```python
from build123d import *

# Parameters (mm, degrees)
ESBO_O1_W                = 72
ESBO_O1_H                = 110
RESSALTO_EXTRUS_O1_DEPTH = 5
ESBO_O2_W                = 51
ESBO_O2_H                = 72
CORTE_EXTRUS_O1_DEPTH    = 4
CHANFRO1_SIZE            = 1.5
CHANFRO1_SIZE_2          = 4
CORTE_EXTRUS_O2_DEPTH    = 66.924198895
CORTE_EXTRUS_O3_DEPTH    = 66.924198895
CORTE_EXTRUS_O4_DEPTH    = 3
CORTE_EXTRUS_O5_DEPTH    = 3
ESBO_O7_W                = 31
ESBO_O7_H                = 44
RESSALTO_EXTRUS_O2_DEPTH = 17
ESBO_O8_W                = 28
ESBO_O8_H                = 42
CORTE_EXTRUS_O6_DEPTH    = 70.318107302
ESBO_O9_W                = 3
ESBO_O9_H                = 1
RESSALTO_EXTRUS_O3_DEPTH = 10
FILETE1_R                = 2


with BuildPart() as part:
    # Esboço1 → Ressalto-extrusão1 (new body)
    with BuildSketch(Plane.XY):
        Rectangle(ESBO_O1_W, ESBO_O1_H)
    extrude(amount=RESSALTO_EXTRUS_O1_DEPTH)

    # Esboço2 → Corte-extrusão1 (cut)
    with BuildSketch(Plane.XY.offset(5)):
        Rectangle(ESBO_O2_W, ESBO_O2_H)
    extrude(amount=-CORTE_EXTRUS_O1_DEPTH, mode=Mode.SUBTRACT)

    # Chanfro1
    # the kernel refuses this chamfer: 4, 1.5 mm, written as the material it takes off along each edge
    with BuildSketch(Plane(origin=(-25.5, -36, 5), x_dir=(0, -0.9953980532473654, 0.09582648689874358), z_dir=(1, 0, 0))) as chanfro1_piece_1_section:
        Polygon((CHANFRO1_SIZE * 0.995398053247, CHANFRO1_SIZE * 0.0958264868987), (-CHANFRO1_SIZE_2 * 0.0958264868987, CHANFRO1_SIZE_2 * 0.995398053247), (0, 0), align=None)
    chanfro1_piece_1 = extrude(amount=51, mode=Mode.PRIVATE)
    chanfro1_piece_1 = split(chanfro1_piece_1, bisect_by=Plane(origin=(0, -36.465264147, 1), z_dir=(0, 0, 1)), keep=Keep.TOP, mode=Mode.PRIVATE)
    add(chanfro1_piece_1, mode=Mode.SUBTRACT)
    with BuildSketch(Plane(origin=(-25.5, 36, 5), x_dir=(-0.9953980532473654, 0, 0.09582648689874379), z_dir=(0, -1, 0))) as chanfro1_piece_2_section:
        Polygon((CHANFRO1_SIZE * 0.995398053247, CHANFRO1_SIZE * 0.0958264868987), (-CHANFRO1_SIZE_2 * 0.0958264868987, CHANFRO1_SIZE_2 * 0.995398053247), (0, 0), align=None)
    chanfro1_piece_2 = extrude(amount=72, mode=Mode.PRIVATE)
    chanfro1_piece_2 = split(chanfro1_piece_2, bisect_by=Plane(origin=(-25.965264147, 0, 1), z_dir=(0, 0, 1)), keep=Keep.TOP, mode=Mode.PRIVATE)
    add(chanfro1_piece_2, mode=Mode.SUBTRACT)
    with BuildSketch(Plane(origin=(25.5, -36, 5), x_dir=(0.9953980532473654, 0, 0.09582648689874379), z_dir=(0, 1, 0))) as chanfro1_piece_3_section:
        Polygon((CHANFRO1_SIZE * 0.995398053247, CHANFRO1_SIZE * 0.0958264868987), (-CHANFRO1_SIZE_2 * 0.0958264868987, CHANFRO1_SIZE_2 * 0.995398053247), (0, 0), align=None)
    chanfro1_piece_3 = extrude(amount=72, mode=Mode.PRIVATE)
    chanfro1_piece_3 = split(chanfro1_piece_3, bisect_by=Plane(origin=(25.965264147, 0, 1), z_dir=(0, 0, 1)), keep=Keep.TOP, mode=Mode.PRIVATE)
    add(chanfro1_piece_3, mode=Mode.SUBTRACT)
    with BuildSketch(Plane(origin=(25.5, 36, 5), x_dir=(0, 0.9953980532473654, 0.09582648689874358), z_dir=(-1, 0, 0))) as chanfro1_piece_4_section:
        Polygon((CHANFRO1_SIZE * 0.995398053247, CHANFRO1_SIZE * 0.0958264868987), (-CHANFRO1_SIZE_2 * 0.0958264868987, CHANFRO1_SIZE_2 * 0.995398053247), (0, 0), align=None)
    chanfro1_piece_4 = extrude(amount=51, mode=Mode.PRIVATE)
    chanfro1_piece_4 = split(chanfro1_piece_4, bisect_by=Plane(origin=(0, 36.465264147, 1), z_dir=(0, 0, 1)), keep=Keep.TOP, mode=Mode.PRIVATE)
    add(chanfro1_piece_4, mode=Mode.SUBTRACT)
    with BuildSketch(Plane(origin=(-35.875482322, -36, 5), x_dir=(0, -0.9953980532473654, 0.09582648689874358), z_dir=(1, 0, 0))) as chanfro1_piece_5a_section:
        Polygon((CHANFRO1_SIZE * 0.995398053247, CHANFRO1_SIZE * 0.0958264868987), (-CHANFRO1_SIZE_2 * 0.0958264868987, CHANFRO1_SIZE_2 * 0.995398053247), (0, 0), align=None)
    chanfro1_piece_5a = extrude(amount=61.375482322, mode=Mode.PRIVATE)
    chanfro1_piece_5a = split(chanfro1_piece_5a, bisect_by=Plane(origin=(-25.5, -36.465264147, 3.645492171), z_dir=(-1, 0, 0)), keep=Keep.TOP, mode=Mode.PRIVATE)
    chanfro1_piece_5a = split(chanfro1_piece_5a, bisect_by=Plane(origin=(-30.687741161, -36.465264147, 1), z_dir=(0, 0, 1)), keep=Keep.TOP, mode=Mode.PRIVATE)
    with BuildSketch(Plane(origin=(-25.5, 36, 5), x_dir=(-0.9953980532473654, 0, 0.09582648689874379), z_dir=(0, -1, 0))) as chanfro1_piece_5b_section:
        Polygon((CHANFRO1_SIZE * 0.995398053247, CHANFRO1_SIZE * 0.0958264868987), (-CHANFRO1_SIZE_2 * 0.0958264868987, CHANFRO1_SIZE_2 * 0.995398053247), (0, 0), align=None)
    chanfro1_piece_5b = extrude(amount=82.375482322, mode=Mode.PRIVATE)
    chanfro1_piece_5b = split(chanfro1_piece_5b, bisect_by=Plane(origin=(-25.965264147, -36, 3.645492171), z_dir=(0, -1, 0)), keep=Keep.TOP, mode=Mode.PRIVATE)
    chanfro1_piece_5b = split(chanfro1_piece_5b, bisect_by=Plane(origin=(-25.965264147, -41.187741161, 1), z_dir=(0, 0, 1)), keep=Keep.TOP, mode=Mode.PRIVATE)
    chanfro1_piece_5 = chanfro1_piece_5a & chanfro1_piece_5b
    add(chanfro1_piece_5, mode=Mode.SUBTRACT)
    with BuildSketch(Plane(origin=(-25.5, -36, 5), x_dir=(0, -0.9953980532473654, 0.09582648689874358), z_dir=(1, 0, 0))) as chanfro1_piece_6a_section:
        Polygon((CHANFRO1_SIZE * 0.995398053247, CHANFRO1_SIZE * 0.0958264868987), (-CHANFRO1_SIZE_2 * 0.0958264868987, CHANFRO1_SIZE_2 * 0.995398053247), (0, 0), align=None)
    chanfro1_piece_6a = extrude(amount=61.375482322, mode=Mode.PRIVATE)
    chanfro1_piece_6a = split(chanfro1_piece_6a, bisect_by=Plane(origin=(25.5, -36.465264147, 3.645492171), z_dir=(1, 0, 0)), keep=Keep.TOP, mode=Mode.PRIVATE)
    chanfro1_piece_6a = split(chanfro1_piece_6a, bisect_by=Plane(origin=(30.687741161, -36.465264147, 1), z_dir=(0, 0, 1)), keep=Keep.TOP, mode=Mode.PRIVATE)
    with BuildSketch(Plane(origin=(25.5, -46.375482322, 5), x_dir=(0.9953980532473654, 0, 0.09582648689874379), z_dir=(0, 1, 0))) as chanfro1_piece_6b_section:
        Polygon((CHANFRO1_SIZE * 0.995398053247, CHANFRO1_SIZE * 0.0958264868987), (-CHANFRO1_SIZE_2 * 0.0958264868987, CHANFRO1_SIZE_2 * 0.995398053247), (0, 0), align=None)
    chanfro1_piece_6b = extrude(amount=82.375482322, mode=Mode.PRIVATE)
    chanfro1_piece_6b = split(chanfro1_piece_6b, bisect_by=Plane(origin=(25.965264147, -36, 3.645492171), z_dir=(0, -1, 0)), keep=Keep.TOP, mode=Mode.PRIVATE)
    chanfro1_piece_6b = split(chanfro1_piece_6b, bisect_by=Plane(origin=(25.965264147, -41.187741161, 1), z_dir=(0, 0, 1)), keep=Keep.TOP, mode=Mode.PRIVATE)
    chanfro1_piece_6 = chanfro1_piece_6a & chanfro1_piece_6b
    add(chanfro1_piece_6, mode=Mode.SUBTRACT)
    with BuildSketch(Plane(origin=(25.5, 36, 5), x_dir=(0, 0.9953980532473654, 0.09582648689874358), z_dir=(-1, 0, 0))) as chanfro1_piece_7a_section:
        Polygon((CHANFRO1_SIZE * 0.995398053247, CHANFRO1_SIZE * 0.0958264868987), (-CHANFRO1_SIZE_2 * 0.0958264868987, CHANFRO1_SIZE_2 * 0.995398053247), (0, 0), align=None)
    chanfro1_piece_7a = extrude(amount=61.375482322, mode=Mode.PRIVATE)
    chanfro1_piece_7a = split(chanfro1_piece_7a, bisect_by=Plane(origin=(-25.5, 36.465264147, 3.645492171), z_dir=(-1, 0, 0)), keep=Keep.TOP, mode=Mode.PRIVATE)
    chanfro1_piece_7a = split(chanfro1_piece_7a, bisect_by=Plane(origin=(-30.687741161, 36.465264147, 1), z_dir=(0, 0, 1)), keep=Keep.TOP, mode=Mode.PRIVATE)
    with BuildSketch(Plane(origin=(-25.5, 46.375482322, 5), x_dir=(-0.9953980532473654, 0, 0.09582648689874379), z_dir=(0, -1, 0))) as chanfro1_piece_7b_section:
        Polygon((CHANFRO1_SIZE * 0.995398053247, CHANFRO1_SIZE * 0.0958264868987), (-CHANFRO1_SIZE_2 * 0.0958264868987, CHANFRO1_SIZE_2 * 0.995398053247), (0, 0), align=None)
    chanfro1_piece_7b = extrude(amount=82.375482322, mode=Mode.PRIVATE)
    chanfro1_piece_7b = split(chanfro1_piece_7b, bisect_by=Plane(origin=(-25.965264147, 36, 3.645492171), z_dir=(0, 1, 0)), keep=Keep.TOP, mode=Mode.PRIVATE)
    chanfro1_piece_7b = split(chanfro1_piece_7b, bisect_by=Plane(origin=(-25.965264147, 41.187741161, 1), z_dir=(0, 0, 1)), keep=Keep.TOP, mode=Mode.PRIVATE)
    chanfro1_piece_7 = chanfro1_piece_7a & chanfro1_piece_7b
    add(chanfro1_piece_7, mode=Mode.SUBTRACT)
    with BuildSketch(Plane(origin=(25.5, -36, 5), x_dir=(0.9953980532473654, 0, 0.09582648689874379), z_dir=(0, 1, 0))) as chanfro1_piece_8a_section:
        Polygon((CHANFRO1_SIZE * 0.995398053247, CHANFRO1_SIZE * 0.0958264868987), (-CHANFRO1_SIZE_2 * 0.0958264868987, CHANFRO1_SIZE_2 * 0.995398053247), (0, 0), align=None)
    chanfro1_piece_8a = extrude(amount=82.375482322, mode=Mode.PRIVATE)
    chanfro1_piece_8a = split(chanfro1_piece_8a, bisect_by=Plane(origin=(25.965264147, 36, 3.645492171), z_dir=(0, 1, 0)), keep=Keep.TOP, mode=Mode.PRIVATE)
    chanfro1_piece_8a = split(chanfro1_piece_8a, bisect_by=Plane(origin=(25.965264147, 41.187741161, 1), z_dir=(0, 0, 1)), keep=Keep.TOP, mode=Mode.PRIVATE)
    with BuildSketch(Plane(origin=(35.875482322, 36, 5), x_dir=(0, 0.9953980532473654, 0.09582648689874358), z_dir=(-1, 0, 0))) as chanfro1_piece_8b_section:
        Polygon((CHANFRO1_SIZE * 0.995398053247, CHANFRO1_SIZE * 0.0958264868987), (-CHANFRO1_SIZE_2 * 0.0958264868987, CHANFRO1_SIZE_2 * 0.995398053247), (0, 0), align=None)
    chanfro1_piece_8b = extrude(amount=61.375482322, mode=Mode.PRIVATE)
    chanfro1_piece_8b = split(chanfro1_piece_8b, bisect_by=Plane(origin=(25.5, 36.465264147, 3.645492171), z_dir=(1, 0, 0)), keep=Keep.TOP, mode=Mode.PRIVATE)
    chanfro1_piece_8b = split(chanfro1_piece_8b, bisect_by=Plane(origin=(30.687741161, 36.465264147, 1), z_dir=(0, 0, 1)), keep=Keep.TOP, mode=Mode.PRIVATE)
    chanfro1_piece_8 = chanfro1_piece_8a & chanfro1_piece_8b
    add(chanfro1_piece_8, mode=Mode.SUBTRACT)

    # Esboço3 → Corte-extrusão2 (cut, through all)
    with BuildSketch(Plane.XY.offset(5)):
        with BuildLine():
            Line((-2, 45), (-2, 39))
            ThreePointArc((-2, 39), (0, 37), (2, 39))
            Line((2, 39), (2, 45))
            ThreePointArc((2, 45), (0, 47), (-2, 45))
        make_face()
    extrude(amount=-CORTE_EXTRUS_O2_DEPTH, mode=Mode.SUBTRACT)

    # Esboço4 → Corte-extrusão3 (cut, through all)
    with BuildSketch(Plane.XY.offset(5)):
        with BuildLine():
            Line((-3, -40), (3, -40))
            ThreePointArc((3, -40), (5, -42), (3, -44))
            Line((3, -44), (-3, -44))
            ThreePointArc((-3, -44), (-5, -42), (-3, -40))
        make_face()
    extrude(amount=-CORTE_EXTRUS_O3_DEPTH, mode=Mode.SUBTRACT)

    # Esboço5 → Corte-extrusão4 (cut)
    with BuildSketch(Plane.XY.offset(5)):
        with BuildLine():
            Line((4.5, 39), (4.5, 45))
            ThreePointArc((4.5, 45), (0, 49.5), (-4.5, 45))
            Line((-4.5, 45), (-4.5, 39))
            ThreePointArc((-4.5, 39), (-4.101470225, 37.148529775), (-2.976470225, 35.625))
            ThreePointArc((-2.976470225, 35.625), (0, 34.5), (2.976470225, 35.625))
            ThreePointArc((2.976470225, 35.625), (4.101470225, 37.148529775), (4.5, 39))
        make_face()
    extrude(amount=-CORTE_EXTRUS_O4_DEPTH, mode=Mode.SUBTRACT)

    # Esboço6 → Corte-extrusão5 (cut)
    with BuildSketch(Plane.XY.offset(5)):
        with BuildLine():
            Line((-3, -46.5), (3, -46.5))
            ThreePointArc((3, -46.5), (7.5, -42), (3, -37.5))
            Line((3, -37.5), (-3, -37.5))
            ThreePointArc((-3, -37.5), (-7.5, -42), (-3, -46.5))
        make_face()
    extrude(amount=-CORTE_EXTRUS_O5_DEPTH, mode=Mode.SUBTRACT)

    # Esboço7 → Ressalto-extrusão2 (add)
    with BuildSketch(Plane(origin=(0, 0, 0), x_dir=(-1, 0, 0), z_dir=(0, 0, -1))):
        Rectangle(ESBO_O7_W, ESBO_O7_H)
    extrude(amount=RESSALTO_EXTRUS_O2_DEPTH)

    # Esboço8 → Corte-extrusão6 (cut, through all)
    with BuildSketch(Plane(origin=(0, 0, -17), x_dir=(-1, 0, 0), z_dir=(0, 0, -1))):
        Rectangle(ESBO_O8_W, ESBO_O8_H)
    extrude(amount=-CORTE_EXTRUS_O6_DEPTH, mode=Mode.SUBTRACT)

    # Esboço9 → Ressalto-extrusão3 (add)
    with BuildSketch(Plane.XY.offset(1)):
        with Locations((-12.5, 10.5)):
            Rectangle(ESBO_O9_W, ESBO_O9_H)
        with Locations((12.5, 10.5)):
            Rectangle(ESBO_O9_W, ESBO_O9_H)
        with Locations((12.5, -10.5)):
            Rectangle(ESBO_O9_W, ESBO_O9_H)
        with Locations((-12.5, -10.5)):
            Rectangle(ESBO_O9_W, ESBO_O9_H)
    extrude(amount=-RESSALTO_EXTRUS_O3_DEPTH)

    # Filete1
    filete1_edges = [part.edges().sort_by_distance(p)[0] for p in [
        (-11, 10.5, 1),
        (11, 10.5, 1),
        (11, -10.5, 1),
        (-11, -10.5, 1),
    ]]
    fillet(filete1_edges, radius=FILETE1_R)


solid = part.part
```
The listing builds one solid part. Answer for the finished solid, in the listing's coordinates (mm). A direction names the side the tool comes from. Coordinates: 2 decimals unless noted, no trailing zeros. Write each loop counter-clockwise with the first axis right and the second up, starting at its lowest first coordinate (ties: lowest second). Pieces come first, ordered by that corner, then holes.
Q1. Section B-B, the plane x = -19.5 is taken. Write down the section's boundary in (y, z).
Returned:
outline: (-55, 0) - (55, 0) - (55, 5) - (37.5, 5) - (36, 1) - (-36, 1) - (-37.5, 5) - (-55, 5) - close
Q2. Which of the six approach directions +Z, -Z, +X, -X, +Y, -Y give full straight-line access (tool end or side, diameter ignored) to faces 4 (the flat face through (0, -39, 2)), 5 (the flat face through (12, -11, -4))?
Returned:
face 4: +Z
face 5: +Z, -Z
Q3. Section C-C, the plane y = -33.5 is taken. Write down the section's boundary in (x, z).
Returned:
outline: (-36, 0) - (36, 0) - (36, 5) - (27, 5) - (25.5, 1) - (-25.5, 1) - (-27, 5) - (-36, 5) - close
Q4. The mould has two halves that part along X. Classify faces 1 (the flat face through (-1, 55, 2)), 2 (the flat face through (-15.5, 0, -8)), 3 (the flat face through (-2, 42, 1)): released by +X, released by -X, zero draft, split by the parting line, or undercut.
Returned:
face 1: zero draft
face 2: released by -X
face 3: undercut
Q5. Given P1, Ø2.5, axis at x = 12.5, z = -1.5, coming from the +Y side; P2, Ø5, axis at y = 3, z = -10.5, coming from the +X side; P3, Ø5, axis at x = -0.5, z = -8, coming from the -Y side, each flat-ended and moving along its own axis, determine where each tip first touches the part or whether it passes through.
Returned:
P1: stops at y = 22
P2: stops at x = 15.5
P3: stops at y = -22
Q6. Find the intervals of material crossed by line 1 along Y through (x, z) = (-1, -0.25); line 2 along X through (y, z) = (5.5, -1); line 3 along Y through (x, z) = (3.5, 2.75), in increasing order.
Returned:
line 1: y = -22 to -21, 21 to 22
line 2: x = -15.5 to -14, 14 to 15.5
line 3: y = -55 to -46.47, -37.53 to -36.66, 47.83 to 55
Q7. Section A-A, the plane y = 16 is taken. Write down the section's boundary in (x, z).
Returned:
outline: (-36, 0) - (-15.5, 0) - (-15.5, -17) - (-14, -17) - (-14, 1) - (-25.5, 1) - (-27, 5) - (-36, 5) - close; (14, -17) - (15.5, -17) - (15.5, 0) - (36, 0) - (36, 5) - (27, 5) - (25.5, 1) - (14, 1) - close
